Check sheet for the modelled part. Datum: model origin and axes. Units: mm. Give positions to 0.01 mm unless a question says otherwise; leave off trailing zeros. Order: outer loops, then holes, each group sorted by start corner. A loop starts at its lowest first (then second) coordinate and runs counter-clockwise, first axis right, second up. Notation, with made-up numbers: (21.5, 11.25) - (32.5, 11.25) arc R11 ccw to (32.5, 21.25) - close; hole circle Ø4 at (3.5, -30). An arc over 180 degrees is marked (long way). Answer in a Markdown table with one row per item.
from build123d import *

# Parameters (mm, degrees)
SKETCH1_W           = 6.35
SKETCH1_H           = 76.2
BOSS_EXTRUDE1_DEPTH = 6.35


with BuildPart() as part:
    # Sketch1 → Boss-Extrude1 (new body)
    with BuildSketch(Plane.XY):
        Polygon((119.544333082, -48.615768355), (94.144333082, -48.615768355), (94.144333082, -42.265768355), (17.944333082, -42.265768355), (17.944333082, -48.615768355), (5.244333082, -48.615768355), (-7.455666918, -48.615768355), (-7.455666918, -42.265768355), (-83.655666918, -42.265768355), (-83.655666918, -48.615768355), (-109.055666918, -48.615768355), (-109.055666918, 179.984231645), (119.544333082, 179.984231645), align=None)
        with Locations((-112.230666918, 72.034231645)):
            Rectangle(SKETCH1_W, SKETCH1_H)
        with Locations((122.719333082, 72.034231645)):
            Rectangle(SKETCH1_W, SKETCH1_H)
    extrude(amount=BOSS_EXTRUDE1_DEPTH)


solid = part.part
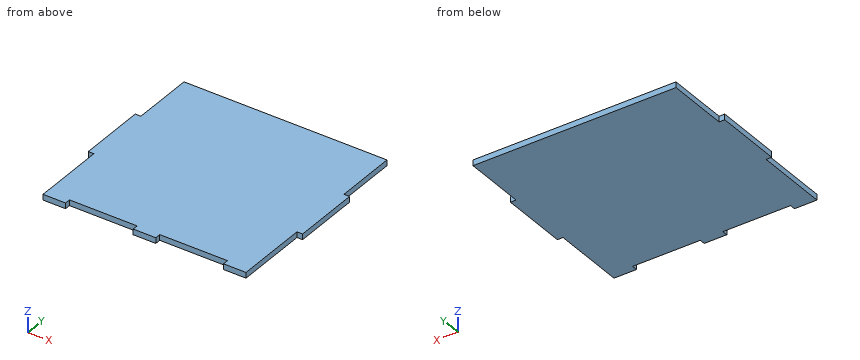
(1) Thickness scan on L1, parallel to Y at x = 77, z = 1.25; L2, parallel to X at y = -29.5, z = 3.25. Record the ranges inside material, lowest first.
Geometry says:
| item | result |
|---|---|
| L1 | -42.27 to 179.98 |
| L2 | -109.06 to 119.54 |
(2) Cross-section at C-C, the plane x = -19. Record the cut outline in (y, z).
Geometry says:
| item | result |
|---|---|
| outline | (-42.27, 0) - (179.98, 0) - (179.98, 6.35) - (-42.27, 6.35) - close |
(3) Cross-section at B-B, the plane y = -4.5. Record the cut outline in (x, z).
Geometry says:
| item | result |
|---|---|
| outline | (-109.06, 0) - (119.54, 0) - (119.54, 6.35) - (-109.06, 6.35) - close |
(4) Cross-section at A-A, the plane z = 4.75. Record the cut outline in (x, y).
Geometry says:
| item | result |
|---|---|
| outline | (-115.41, 33.93) - (-109.06, 33.93) - (-109.06, -48.62) - (-83.66, -48.62) - (-83.66, -42.27) - (-7.46, -42.27) - (-7.46, -48.62) - (17.94, -48.62) - (17.94, -42.27) - (94.14, -42.27) - (94.14, -48.62) - (119.54, -48.62) - (119.54, 33.93) - (125.89, 33.93) - (125.89, 110.13) - (119.54, 110.13) - (119.54, 179.98) - (-109.06, 179.98) - (-109.06, 110.13) - (-115.41, 110.13) - close |
(5) Gauge pin test, flat ends, axial feed: P1, Ø2, axis at y = 125, z = 5, coming from the -X side; P2, Ø1.9, axis at y = 151.5, z = 2.5, coming from the +X side; P3, Ø1.5, axis at x = 89, z = 2.5, coming from the -Y side. Record the tip position at first contact, or that the pin passes through.
Geometry says:
| item | result |
|---|---|
| P1 | x = -109.06 |
| P2 | x = 119.54 |
| P3 | y = -42.27 |
